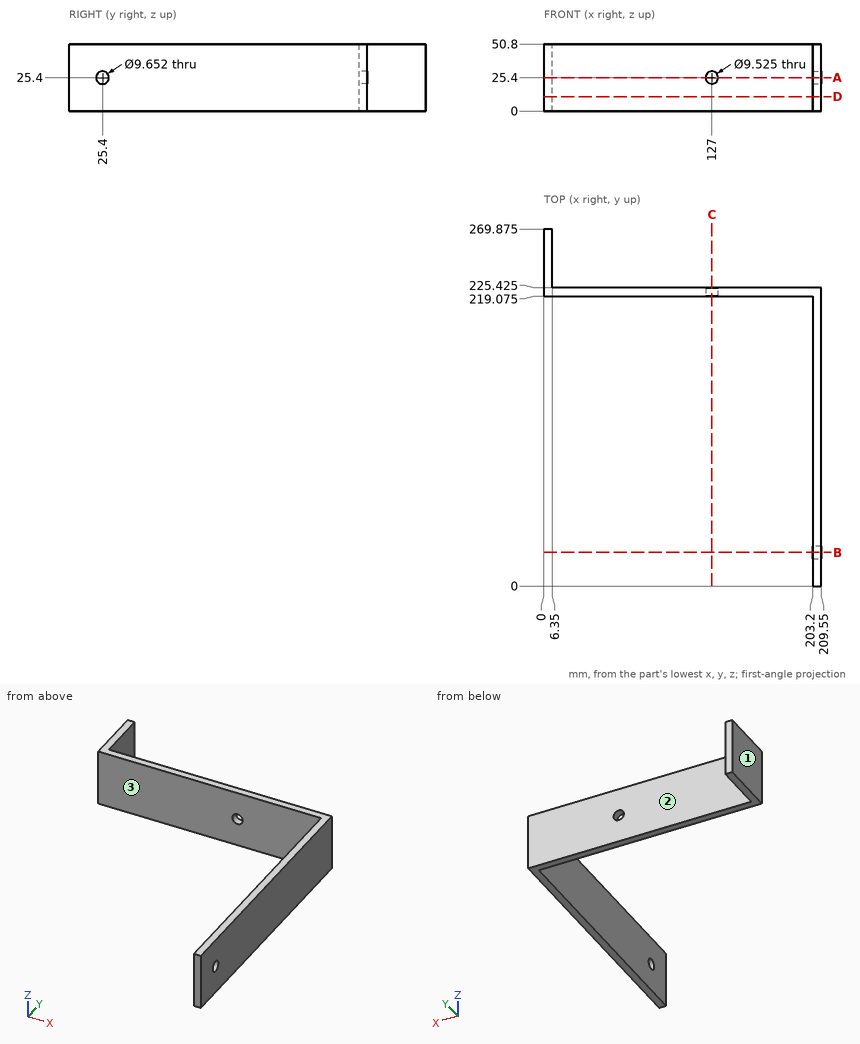
Geometry: see drawing. Coordinates: mm, zero at the bounding-box minimum. A direction names the side the tool comes from. Give positions to 0.01 mm unless a question says otherwise; leave off trailing zeros. Loops run counter-clockwise (first coordinate to the right, second up) from the corner with the lowest first, then second, coordinate; pieces in that order, holes last. Notation, with made-up numbers: (54, -17) - (58, -17) arc R20 ccw to (58, 3) - close; hole circle Ø2 at (-34.75, 8.25). An arc over 180 degrees is marked (long way). One line per question, with ' | ' between items. Start each with the question number.
(1) Section query B-B on y = 25.4. Return loops of the section in (x, z).
(2) Contact query for flat-ended pins moving along their axis: pin 1 (3 mm diameter, centred on y = 210.5, z = 43.5, fed in from -X); pin 2 (10 mm diameter, centred on x = 88, z = 21.5, fed in from -Y) (3 decimals); pin 3 (15 mm diameter, centred on x = 104.5, z = 37.5, fed in from +Y) (3 decimals). Output: stop coordinate, or through.
(3) Section query D-D on z = 11. Return loops of the section in (x, y) (3 decimals), then the cut area to 3 significant figures.
(4) Section query C-C on x = 127. Return loops of the section in (y, z) (1 decimal).
(5) Ray query, line 1 (Z direction, x = 206, y = 25); line 2 (X direction, y = 224, z = 25); line 3 (Y direction, x = 62, z = 9) (3 decimals). Return the intervals inside material, ascending. Write a range as from..to.
(6) Section query A-A on z = 25.4. Count the separate pieces of the cut face and the enclosed holes in it, then the cut area to 3 significant figures.
(7) Reachability of the marked faces 1, 2 and 3 from +Z, -Z, +X, -X, +Y, -Y: full face, straight path, thin tool, end or side. Return the list, or none.
The answers:
1) outline: (203.2, 0) - (209.55, 0) - (209.55, 20.57) - (203.2, 20.57) - close; (203.2, 30.23) - (209.55, 30.23) - (209.55, 50.8) - (203.2, 50.8) - close
2) pin 1: x = 203.2 | pin 2: y = 219.075 | pin 3: y = 225.425
3) outline: (0, 219.075) - (203.2, 219.075) - (203.2, 0) - (209.55, 0) - (209.55, 225.425) - (6.35, 225.425) - (6.35, 269.875) - (0, 269.875) - close | area: 3,000 mm2
4) outline: (219.1, 0) - (225.4, 0) - (225.4, 20.6) - (219.1, 20.6) - close; (219.1, 30.2) - (225.4, 30.2) - (225.4, 50.8) - (219.1, 50.8) - close
5) line 1: 0..20.59, 30.21..50.8 | line 2: 0..122.25, 131.75..209.55 | line 3: 219.075..225.425
6) separate pieces: 3 | enclosed holes: 0 | area: 2,880 mm2
7) face 1: +Z, -Z, -X, +Y, -Y | face 2: +Z, -Z, +X, +Y | face 3: +Z, -Z, -X, -Y
